```python
from build123d import *

# Parameters (mm, degrees)
BOSS_EXTRUDE1_DEPTH = 2.4


with BuildPart() as part:
    # Sketch1 → Boss-Extrude1 (new body)
    with BuildSketch(Plane.XY):
        Polygon((0, 3.175426481), (-2.75, 1.58771324), (-2.75, -1.58771324), (0, -3.175426481), (2.75, -1.58771324), (2.75, 1.58771324), align=None)
    extrude(amount=-BOSS_EXTRUDE1_DEPTH)

    # Sketch4 → Cut-Revolve1 (revolve, cut)
    with BuildSketch(Plane(origin=(0, 0, 0), x_dir=(0, 0, -1), z_dir=(1, 0, 0))):
        Polygon((2.4, 3.175426481), (1.865704772, 3.175426481), (2.4, 2.25), align=None)
        Polygon((0, 3.175426481), (0.534295228, 3.175426481), (0, 2.25), align=None)
    revolve(axis=Axis((0, 0, 0), (0, 0, -1)), mode=Mode.SUBTRACT)

    # Sketch5 → Cut-Revolve2 (revolve, cut)
    with BuildSketch(Plane(origin=(0, 0, 0), x_dir=(0, 0, -1), z_dir=(1, 0, 0))):
        Polygon((0, 0), (0, 1.55), (0.173205081, 1.25), (2.226794919, 1.25), (2.4, 1.55), (2.4, 0), align=None)
    revolve(axis=Axis((0, 0, 0), (0, 0, -1)), mode=Mode.SUBTRACT)


solid = part.part
```
Input: part model. Units: mm. Frame: model coordinates. Coordinates: 2 decimals unless noted, no trailing zeros. Loops run counter-clockwise (first coordinate to the right, second up) from the corner with the lowest first, then second, coordinate; pieces in that order, holes last. Notation, with made-up numbers: M -40,-33.5 L -3,-33.5 A21 cw -3,-25.5 Z; hole C -19.75,35 d5. An arc over 180 degrees is marked long. Use a Markdown table: item, result. Add a question column.
1) Section A-A, the plane y = 0. Return the cut outline in (x, z).
2) Draft query along Y for faces 1 (the flat face through (1.394, 2.37, -1.187)), 2 (the flat face through (1.36, -2.39, -1.19)), 3 (the flat face through (-2, 0, -2.4)), 4 (the cylindrical face through (-1.22, -0.27, -1.21)). Return one class per face: +Y half, -Y half, draft (parallel to the pull), parting line (faces both ways), or undercut.
3) Section B-B, the plane z = -0.8. Return the cut outline in (x, y).
4) Line query: L1, parallel to X at y = 0, z = -1; L2, parallel to Y at x = -0.65, z = -0.8; L3, parallel to X at y = -1, z = -1.6. Output: solid intervals per line, ascending. Write a range as from..to.
5) Pin query (flat end, axial travel): P1, Ø1, axis at x = 2, z = -2, coming from the -Y side; P2, Ø3, axis at x = 0, y = 0, coming from the +Z side. Return the tip coordinate at first contact, or that it passes through.
Answer below:
| question | item | result |
|---|---|---|
| 1 | outline | M -2.75,-2.11 L -2.25,-2.4 L -1.55,-2.4 L -1.25,-2.23 L -1.25,-0.17 L -1.55,0 L -2.25,0 L -2.75,-0.29 Z; M 1.25,-2.23 L 1.55,-2.4 L 2.25,-2.4 L 2.75,-2.11 L 2.75,-0.29 L 2.25,0 L 1.55,0 L 1.25,-0.17 Z |
| 2 | face 1 | +Y half |
| 2 | face 2 | -Y half |
| 2 | face 3 | draft |
| 2 | face 4 | undercut |
| 3 | outline | M -2.75,-1.59 L 0,-3.18 L 2.75,-1.59 L 2.75,1.59 L 0,3.18 L -2.75,1.59 Z; hole C 0,0 d2.5 |
| 4 | L1 | -2.75..-1.25, 1.25..2.75 |
| 4 | L2 | -2.8..-1.07, 1.07..2.8 |
| 4 | L3 | -2.75..-0.75, 0.75..2.75 |
| 5 | P1 | y = -2.31 |
| 5 | P2 | z = -0.03 |
